Read the model definition and answer for the solid it produces. Units are mm, in the model's axes. Face numbers are marked on the shaded views. A direction names the side the tool comes from. Coordinates: 2 decimals unless noted, no trailing zeros. Write each loop counter-clockwise with the first axis right and the second up, starting at its lowest first coordinate (ties: lowest second). Pieces come first, ordered by that corner, then holes. Notation, with made-up numbers: (12, -5) - (34, -5) arc R16 cw to (34, 22) - close; hole circle Ø10 at (-25, -40). An arc over 180 degrees is marked (long way). Return JSON: item names as keys, results as strings.
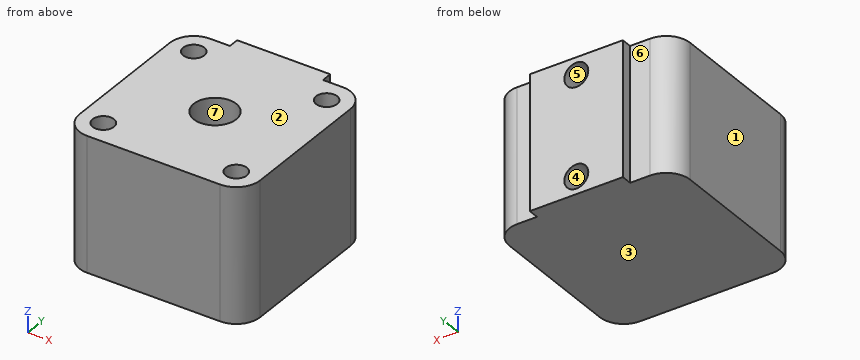
```python
from build123d import *

# Parameters (mm, degrees)
SALIENTE_EXTRUIR1_DEPTH = 50.5
CROQUIS2_R              = 4
CORTAR_EXTRUIR1_DEPTH   = 20
CROQUIS3_R              = 8
CORTAR_EXTRUIR2_DEPTH   = 20
CROQUIS4_R              = 4.5
CORTAR_EXTRUIR3_DEPTH   = 10


with BuildPart() as part:
    # Croquis1 → Saliente-Extruir1 (new body)
    with BuildSketch(Plane.XY):
        with BuildLine():
            Line((-17.5, 34), (-17.5, 38))
            Line((-17.5, 38), (17.5, 38))
            Line((17.5, 38), (17.5, 34))
            Line((17.5, 34), (25, 34))
            ThreePointArc((25, 34), (31.363961031, 31.363961031), (34, 25))
            Line((34, 25), (34, -25))
            ThreePointArc((34, -25), (31.363961031, -31.363961031), (25, -34))
            Line((25, -34), (-25, -34))
            ThreePointArc((-25, -34), (-31.363961031, -31.363961031), (-34, -25))
            Line((-34, -25), (-34, 25))
            ThreePointArc((-34, 25), (-31.363961031, 31.363961031), (-25, 34))
            Line((-25, 34), (-17.5, 34))
        make_face()
    extrude(amount=-SALIENTE_EXTRUIR1_DEPTH)

    # Croquis2 → Cortar-Extruir1 (cut)
    with BuildSketch(Plane.XY):
        with Locations((-25, 25)):
            Circle(CROQUIS2_R)
        with Locations((-25, -25)):
            Circle(CROQUIS2_R)
        with Locations((25, -25)):
            Circle(CROQUIS2_R)
        with Locations((25, 25)):
            Circle(CROQUIS2_R)
    extrude(amount=-CORTAR_EXTRUIR1_DEPTH, mode=Mode.SUBTRACT)

    # Croquis3 → Cortar-Extruir2 (cut)
    with BuildSketch(Plane.XY):
        Circle(CROQUIS3_R)
    extrude(amount=-CORTAR_EXTRUIR2_DEPTH, mode=Mode.SUBTRACT)

    # Croquis4 → Cortar-Extruir3 (cut)
    with BuildSketch(Plane(origin=(0, 38, 0), x_dir=(1, 0, 0), z_dir=(0, 1, 0))):
        with Locations(Location((0, 6.5, 0), (0, 0, 270))):
            Circle(CROQUIS4_R)
        with Locations(Location((0, 44, 0), (0, 0, 270))):
            Circle(CROQUIS4_R)
    extrude(amount=-CORTAR_EXTRUIR3_DEPTH, mode=Mode.SUBTRACT)


solid = part.part
```
(1) Flat-ended cylindrical pins translate along their axes: P1, Ø4, axis at x = 21.5, z = -44.5, coming from the +Y side; P2, Ø1, axis at x = 14.5, y = 4, coming from the +Z side; P3, Ø7, axis at x = -25, y = 25, coming from the +Z side; P4, Ø2, axis at y = 35.5, z = -25.5, coming from the -X side. Find the tip coordinate at first contact, or state that the pin passes through.
Answer:
{"P1": "y = 34", "P2": "z = 0", "P3": "z = -20", "P4": "x = -17.5"}
(2) Which of the six approach directions +Z, -Z, +X, -X, +Y, -Y give full straight-line access (tool end or side, diameter ignored) to the marked faces 5, 6 and 7?
Answer:
{"face 5": "+Y", "face 6": "+Z, -Z, -X, +Y", "face 7": "+Z"}
(3) Straight lines are drawn through the part: line 1 (Y direction, x = -25, z = -9.25); line 2 (Y direction, x = 0, z = -4.75); line 3 (Y direction, x = 21.5, z = -9.5). For each, find the intervals that lie inside material, in ascending order. Write a range as from..to.
Answer:
{"line 1": "-34..-29, -21..21, 29..34", "line 2": "-34..-8, 8..28", "line 3": "-34..-26.94, -23.06..23.06, 26.94..34"}
(4) A cutting plane is placed at A-A (z = -6.5). Determine the outline of the cut face in (x, y).
Answer:
{"outline": "(-34, -25) arc R9 ccw to (-25, -34) - (25, -34) arc R9 ccw to (34, -25) - (34, 25) arc R9 ccw to (25, 34) - (17.5, 34) - (17.5, 38) - (4.5, 38) - (4.5, 28) - (-4.5, 28) - (-4.5, 38) - (-17.5, 38) - (-17.5, 34) - (-25, 34) arc R9 ccw to (-34, 25) - close; hole circle Ø8 at (-25, -25); hole circle Ø8 at (-25, 25); hole circle Ø16 at (0, 0); hole circle Ø8 at (25, -25); hole circle Ø8 at (25, 25)"}
(5) A cutting plane is placed at B-B (x = 0). Determine the outline of the cut face in (y, z), and give its area (3 significant figures).
Answer:
{"outline": "(-34, -50.5) - (38, -50.5) - (38, -48.5) - (28, -48.5) - (28, -39.5) - (38, -39.5) - (38, -11) - (28, -11) - (28, -2) - (38, -2) - (38, 0) - (8, 0) - (8, -20) - (-8, -20) - (-8, 0) - (-34, 0) - close", "area": "3,140 mm²"}
(6) A cutting plane is placed at D-D (y = -28). Determine the outline of the cut face in (x, z).
Answer:
{"outline": "(-33.49, -50.5) - (33.49, -50.5) - (33.49, 0) - (27.65, 0) - (27.65, -20) - (22.35, -20) - (22.35, 0) - (-22.35, 0) - (-22.35, -20) - (-27.65, -20) - (-27.65, 0) - (-33.49, 0) - close"}
(7) Determine the mould class of the marked faces 1, 2, 3 and 4 for opening direction Z: +Z half, -Z half, draft (parallel to the pull), parting line (faces both ways), or undercut.
Answer:
{"face 1": "draft", "face 2": "+Z half", "face 3": "-Z half", "face 4": "undercut"}
(8) A cutting plane is placed at C-C (z = -44). Determine the outline of the cut face in (x, y).
Answer:
{"outline": "(-34, -25) arc R9 ccw to (-25, -34) - (25, -34) arc R9 ccw to (34, -25) - (34, 25) arc R9 ccw to (25, 34) - (17.5, 34) - (17.5, 38) - (4.5, 38) - (4.5, 28) - (-4.5, 28) - (-4.5, 38) - (-17.5, 38) - (-17.5, 34) - (-25, 34) arc R9 ccw to (-34, 25) - close"}
